Geometry check sheet. Reference: the model listing, model coordinates, mm. A direction names the side the tool comes from. Round coordinates to 2 decimals unless told otherwise and drop trailing zeros. Loops run counter-clockwise (first coordinate to the right, second up) from the corner with the lowest first, then second, coordinate; pieces in that order, holes last. Notation, with made-up numbers: (79.5, 35) - (131.5, 35) arc R17 ccw to (131.5, 68) - close; hole circle Ø7 at (46.25, 54). An arc over 180 degrees is marked (long way). Answer in a Markdown table with one row per item. Add a question column.
```python
from build123d import *

# Parameters (mm, degrees)
BASE_EXTRUDE_DEPTH = 203.2
LSLOT_DEPTH        = 225.525158509
LPATTERN1_COUNT    = 2
LPATTERN1_PITCH    = 101.6


with BuildPart() as part:
    # Sketch1 → Base-Extrude (new body)
    with BuildSketch(Plane.XY):
        with BuildLine():
            Line((17.6403, 16.339286512), (19.729882578, 19.063533504))
            ThreePointArc((19.729882578, 19.063533504), (19.156045845, 20.609744632), (17.6403, 21.2598))
            Line((17.6403, 21.2598), (14.70327367, 21.2598))
            ThreePointArc((14.70327367, 21.2598), (13.223883481, 20.647016519), (12.6111, 19.16762633))
            Line((12.6111, 19.16762633), (12.6111, 15.61465))
            Line((12.6111, 15.61465), (11.1125, 15.61465))
            Line((11.1125, 15.61465), (11.1125, 19.16762633))
            ThreePointArc((11.1125, 19.16762633), (12.164213258, 21.706686742), (14.70327367, 22.7584))
            Line((14.70327367, 22.7584), (17.6403, 22.7584))
            ThreePointArc((17.6403, 22.7584), (20.415434554, 21.446284653), (21.162428673, 18.4688666))
            Line((21.162428673, 18.4688666), (19.1389, 15.830735923))
            Line((19.1389, 15.830735923), (19.1389, 10.749129415))
            Line((19.1389, 10.749129415), (20.6375, 9.0662125))
            Line((20.6375, 9.0662125), (20.6375, -4.8244125))
            Line((20.6375, -4.8244125), (19.1389, -6.507329415))
            Line((19.1389, -6.507329415), (19.1389, -13.358784555))
            Line((19.1389, -13.358784555), (20.553458003, -14.773342558))
            ThreePointArc((20.553458003, -14.773342558), (18.729942105, -18.270236732), (15.019825564, -16.932883251))
            ThreePointArc((15.019825564, -16.932883251), (13.000752562, -16.523120627), (12.480559153, -18.5166))
            Line((12.480559153, -18.5166), (-12.480559153, -18.5166))
            ThreePointArc((-12.480559153, -18.5166), (-13.000752562, -16.523120627), (-15.019825564, -16.932883251))
            ThreePointArc((-15.019825564, -16.932883251), (-18.729942105, -18.270236732), (-20.553458003, -14.773342558))
            Line((-20.553458003, -14.773342558), (-19.1389, -13.358784555))
            Line((-19.1389, -13.358784555), (-19.1389, -6.507329415))
            Line((-19.1389, -6.507329415), (-20.6375, -4.8244125))
            Line((-20.6375, -4.8244125), (-20.6375, 9.0662125))
            Line((-20.6375, 9.0662125), (-19.1389, 10.749129415))
            Line((-19.1389, 10.749129415), (-19.1389, 15.830735923))
            Line((-19.1389, 15.830735923), (-21.162428673, 18.4688666))
            ThreePointArc((-21.162428673, 18.4688666), (-20.415434554, 21.446284653), (-17.6403, 22.7584))
            Line((-17.6403, 22.7584), (-14.70327367, 22.7584))
            ThreePointArc((-14.70327367, 22.7584), (-12.164213258, 21.706686742), (-11.1125, 19.16762633))
            Line((-11.1125, 19.16762633), (-11.1125, 15.61465))
            Line((-11.1125, 15.61465), (-12.6111, 15.61465))
            Line((-12.6111, 15.61465), (-12.6111, 19.16762633))
            ThreePointArc((-12.6111, 19.16762633), (-13.223883481, 20.647016519), (-14.70327367, 21.2598))
            Line((-14.70327367, 21.2598), (-17.6403, 21.2598))
            ThreePointArc((-17.6403, 21.2598), (-19.156045845, 20.609744632), (-19.729882578, 19.063533504))
            Line((-19.729882578, 19.063533504), (-17.6403, 16.339286512))
            Line((-17.6403, 16.339286512), (-17.6403, 10.17860201))
            Line((-17.6403, 10.17860201), (-19.1389, 8.495685095))
            Line((-19.1389, 8.495685095), (-19.1389, -4.253885095))
            Line((-19.1389, -4.253885095), (-17.6403, -5.93680201))
            Line((-17.6403, -5.93680201), (-17.6403, -13.979525))
            Line((-17.6403, -13.979525), (-19.1389, -15.478125))
            ThreePointArc((-19.1389, -15.478125), (-18.092238669, -16.906954381), (-16.414285827, -16.33992034))
            ThreePointArc((-16.414285827, -16.33992034), (-13.428073412, -14.819877156), (-10.898992189, -17.018))
            Line((-10.898992189, -17.018), (10.898992189, -17.018))
            ThreePointArc((10.898992189, -17.018), (13.323359075, -14.834630878), (16.30518861, -16.15877141))
            ThreePointArc((16.30518861, -16.15877141), (17.990302879, -16.935279743), (19.1389, -15.478125))
            Line((19.1389, -15.478125), (17.6403, -13.979525))
            Line((17.6403, -13.979525), (17.6403, -5.93680201))
            Line((17.6403, -5.93680201), (19.1389, -4.253885095))
            Line((19.1389, -4.253885095), (19.1389, 8.495685095))
            Line((19.1389, 8.495685095), (17.6403, 10.17860201))
            Line((17.6403, 10.17860201), (17.6403, 16.339286512))
        make_face()
    extrude(amount=BASE_EXTRUDE_DEPTH)

    # Sketch2 → LSlot (cut, through all)
    with BuildSketch(Plane(origin=(-0.093451067, -18.5166, -16.466077999), x_dir=(1, 0, 0), z_dir=(0, -1, 0))):
        with BuildLine():
            Line((5.252826067, 95.047327999), (5.252826067, 29.166077999))
            ThreePointArc((5.252826067, 29.166077999), (0.093451067, 24.006702999), (-5.065923933, 29.166077999))
            Line((-5.065923933, 29.166077999), (-5.065923933, 95.047327999))
            ThreePointArc((-5.065923933, 95.047327999), (0.093451067, 100.206702999), (5.252826067, 95.047327999))
        make_face()
    lslot = extrude(amount=-LSLOT_DEPTH, mode=Mode.SUBTRACT)

    # LPattern1: LSlot ×2
    with Locations(*[(0, 0, i * LPATTERN1_PITCH) for i in range(1, LPATTERN1_COUNT)]):
        add(lslot, mode=Mode.SUBTRACT)


solid = part.part
```
Q1. Set-up check for faces 1 (the flat face through (-19.139, 2, 100)), 2 (the flat face through (19.139, 13, 100)), 3 (the cylindrical face through (0.11, -17.78, 7.54)), 4 (the flat face through (-20.638, 2, 100)), 5 (the flat face through (20.638, 2, 100)): record each of +Z, -Z, +X, -X, +Y, -Y from which the full face is reachable in a straight line by a thin tool's end or side.
Q2. Cross-section at C-C, the plane x = 8. Enter the section's corners in (y, z).
Q3. Cross-section at B-B, the plane x = 0. Enter the section's corners in (y, z).
Q4. Depth check by flat-ended pin: P1, Ø1.5, axis at y = 14.5, z = 132, coming from the +X side; P2, Ø0.7, axis at y = -18, z = 160.5, coming from the -X side; P3, Ø7, axis at y = 14.5, z = 131, coming from the +X side; P4, Ø4, axis at y = 18, z = 106.5, coming from the -X side. Enter the tip coordinate at first touch or a pass-through.
Q5. Cross-section at A-A, the plane y = 13. Enter the section's corners in (x, z), plus the area to 3 significant figures.
Q6. Release check for a two-part mould opening along Y. For faces 6 (the flat face through (11.112, 17, 100)), 7 (the flat face through (-12.611, 17, 100)), 8 (the flat face through (-19.139, 13, 100)), 9 (the cylindrical face through (-12.19, 21.73, 100.18)) record: +Y half, -Y half, draft (parallel to the pull), parting line (faces both ways), or undercut.
Q7. Scan lines: line 1 (X direction, y = -10.5, z = 24); line 2 (X direction, y = -1, z = 171); line 3 (Y direction, x = -19, z = 101). Record each from-to range of solid material in increasing order. Write a range as from..to.
Check sheet entries:
| question | item | result |
|---|---|---|
| 1 | face 1 | +Z, -Z |
| 1 | face 2 | +Z, -Z, +X |
| 1 | face 3 | +Y, -Y |
| 1 | face 4 | +Z, -Z, -X, -Y |
| 1 | face 5 | +Z, -Z, +X, -Y |
| 2 | outline | (-18.52, 0) - (-17.02, 0) - (-17.02, 203.2) - (-18.52, 203.2) - close |
| 3 | outline | (-18.52, 0) - (-17.02, 0) - (-17.02, 7.54) - (-18.52, 7.54) - close; (-18.52, 83.74) - (-17.02, 83.74) - (-17.02, 109.14) - (-18.52, 109.14) - close; (-18.52, 185.34) - (-17.02, 185.34) - (-17.02, 203.2) - (-18.52, 203.2) - close |
| 4 | P1 | x = 19.14 |
| 4 | P2 | x = -19.71 |
| 4 | P3 | x = 20.8 |
| 4 | P4 | x = -21.23 |
| 5 | outline | (-19.14, 0) - (-17.64, 0) - (-17.64, 203.2) - (-19.14, 203.2) - close; (17.64, 0) - (19.14, 0) - (19.14, 203.2) - (17.64, 203.2) - close |
| 5 | area | 609 mm² |
| 6 | face 6 | draft |
| 6 | face 7 | undercut |
| 6 | face 8 | undercut |
| 6 | face 9 | +Y half |
| 7 | line 1 | -19.14..-17.64, 17.64..19.14 |
| 7 | line 2 | -20.64..-19.14, 19.14..20.64 |
| 7 | line 3 | -18.15..-16.11, -15.34..-4.41, 8.65..18.11, 20.76..22.49 |
